from build123d import *

# Parameters (mm, degrees)
SKETCH_1_W      = 29
SKETCH_1_H      = 12.7
EXTRUDE_1_DEPTH = 15.7
EXTRUDE_2_DEPTH = 3.5
FILLET_1_R      = 0.05
CHAMFER_1_SIZE  = 1.5
FILLET_2_R      = 0.75


with BuildPart() as part:
    # Эскиз1 → Бобышка-Вытянуть1 (new body)
    with BuildSketch(Plane(origin=(0, 0, 0), x_dir=(1, 0, 0), z_dir=(0, 1, 0))):
        Rectangle(SKETCH_1_W, SKETCH_1_H)
    extrude(amount=EXTRUDE_1_DEPTH)

    # Эскиз2 → Бобышка-Вытянуть2 (add)
    with BuildSketch(Plane.XZ):
        with BuildLine():
            Line((-12.3, 4.15), (-11.9, 4.15))
            ThreePointArc((-11.9, 4.15), (-11.864644661, 4.135355339), (-11.85, 4.1))
            Line((-11.85, 4.1), (-11.85, 3.4))
            ThreePointArc((-11.85, 3.4), (-11.864644661, 3.364644661), (-11.9, 3.35))
            Line((-11.9, 3.35), (-12.3, 3.35))
            ThreePointArc((-12.3, 3.35), (-12.335355339, 3.364644661), (-12.35, 3.4))
            Line((-12.35, 3.4), (-12.35, 4.1))
            ThreePointArc((-12.35, 4.1), (-12.335355339, 4.135355339), (-12.3, 4.15))
        make_face()
        with BuildLine():
            Line((2.65, 4.1), (2.65, 3.4))
            ThreePointArc((2.65, 3.4), (2.664644661, 3.364644661), (2.7, 3.35))
            Line((2.7, 3.35), (3.1, 3.35))
            ThreePointArc((3.1, 3.35), (3.135355339, 3.364644661), (3.15, 3.4))
            Line((3.15, 3.4), (3.15, 4.1))
            ThreePointArc((3.15, 4.1), (3.135355339, 4.135355339), (3.1, 4.15))
            Line((3.1, 4.15), (2.7, 4.15))
            ThreePointArc((2.7, 4.15), (2.664644661, 4.135355339), (2.65, 4.1))
        make_face()
        with BuildLine():
            Line((7.65, 4.1), (7.65, 3.4))
            ThreePointArc((7.65, 3.4), (7.664644661, 3.364644661), (7.7, 3.35))
            Line((7.7, 3.35), (8.1, 3.35))
            ThreePointArc((8.1, 3.35), (8.135355339, 3.364644661), (8.15, 3.4))
            Line((8.15, 3.4), (8.15, 4.1))
            ThreePointArc((8.15, 4.1), (8.135355339, 4.135355339), (8.1, 4.15))
            Line((8.1, 4.15), (7.7, 4.15))
            ThreePointArc((7.7, 4.15), (7.664644661, 4.135355339), (7.65, 4.1))
        make_face()
        with BuildLine():
            Line((12.65, 4.1), (12.65, 3.4))
            ThreePointArc((12.65, 3.4), (12.664644661, 3.364644661), (12.7, 3.35))
            Line((12.7, 3.35), (13.1, 3.35))
            ThreePointArc((13.1, 3.35), (13.135355339, 3.364644661), (13.15, 3.4))
            Line((13.15, 3.4), (13.15, 4.1))
            ThreePointArc((13.15, 4.1), (13.135355339, 4.135355339), (13.1, 4.15))
            Line((13.1, 4.15), (12.7, 4.15))
            ThreePointArc((12.7, 4.15), (12.664644661, 4.135355339), (12.65, 4.1))
        make_face()
        with BuildLine():
            Line((2.65, -3.4), (2.65, -4.1))
            ThreePointArc((2.65, -4.1), (2.664644661, -4.135355339), (2.7, -4.15))
            Line((2.7, -4.15), (3.1, -4.15))
            ThreePointArc((3.1, -4.15), (3.135355339, -4.135355339), (3.15, -4.1))
            Line((3.15, -4.1), (3.15, -3.4))
            ThreePointArc((3.15, -3.4), (3.135355339, -3.364644661), (3.1, -3.35))
            Line((3.1, -3.35), (2.7, -3.35))
            ThreePointArc((2.7, -3.35), (2.664644661, -3.364644661), (2.65, -3.4))
        make_face()
        with BuildLine():
            Line((7.65, -3.4), (7.65, -4.1))
            ThreePointArc((7.65, -4.1), (7.664644661, -4.135355339), (7.7, -4.15))
            Line((7.7, -4.15), (8.1, -4.15))
            ThreePointArc((8.1, -4.15), (8.135355339, -4.135355339), (8.15, -4.1))
            Line((8.15, -4.1), (8.15, -3.4))
            ThreePointArc((8.15, -3.4), (8.135355339, -3.364644661), (8.1, -3.35))
            Line((8.1, -3.35), (7.7, -3.35))
            ThreePointArc((7.7, -3.35), (7.664644661, -3.364644661), (7.65, -3.4))
        make_face()
        with BuildLine():
            Line((12.65, -3.4), (12.65, -4.1))
            ThreePointArc((12.65, -4.1), (12.664644661, -4.135355339), (12.7, -4.15))
            Line((12.7, -4.15), (13.1, -4.15))
            ThreePointArc((13.1, -4.15), (13.135355339, -4.135355339), (13.15, -4.1))
            Line((13.15, -4.1), (13.15, -3.4))
            ThreePointArc((13.15, -3.4), (13.135355339, -3.364644661), (13.1, -3.35))
            Line((13.1, -3.35), (12.7, -3.35))
            ThreePointArc((12.7, -3.35), (12.664644661, -3.364644661), (12.65, -3.4))
        make_face()
        with BuildLine():
            Line((-12.35, -3.4), (-12.35, -4.1))
            ThreePointArc((-12.35, -4.1), (-12.335355339, -4.135355339), (-12.3, -4.15))
            Line((-12.3, -4.15), (-11.9, -4.15))
            ThreePointArc((-11.9, -4.15), (-11.864644661, -4.135355339), (-11.85, -4.1))
            Line((-11.85, -4.1), (-11.85, -3.4))
            ThreePointArc((-11.85, -3.4), (-11.864644661, -3.364644661), (-11.9, -3.35))
            Line((-11.9, -3.35), (-12.3, -3.35))
            ThreePointArc((-12.3, -3.35), (-12.335355339, -3.364644661), (-12.35, -3.4))
        make_face()
    extrude(amount=EXTRUDE_2_DEPTH)

    # Скругление1
    fillet_1_edges = [part.edges().sort_by_distance(p)[0] for p in [
        (7.664644661, -3.5, -4.135355339),
        (7.9, -3.5, -4.15),
        (8.135355339, -3.5, -4.135355339),
        (8.15, -3.5, -3.75),
        (8.135355339, -3.5, -3.364644661),
        (7.9, -3.5, -3.35),
        (7.664644661, -3.5, -3.364644661),
        (7.65, -3.5, -3.75),
        (12.664644661, -3.5, -4.135355339),
        (12.9, -3.5, -4.15),
        (13.135355339, -3.5, -4.135355339),
        (13.15, -3.5, -3.75),
        (13.135355339, -3.5, -3.364644661),
        (12.9, -3.5, -3.35),
        (12.664644661, -3.5, -3.364644661),
        (12.65, -3.5, -3.75),
        (-12.335355339, -3.5, -4.135355339),
        (-12.1, -3.5, -4.15),
        (-11.864644661, -3.5, -4.135355339),
        (-11.85, -3.5, -3.75),
        (-11.864644661, -3.5, -3.364644661),
        (-12.1, -3.5, -3.35),
        (-12.335355339, -3.5, -3.364644661),
        (-12.35, -3.5, -3.75),
        (-12.335355339, -3.5, 3.364644661),
        (-12.1, -3.5, 3.35),
        (-11.864644661, -3.5, 3.364644661),
        (-11.85, -3.5, 3.75),
        (-11.864644661, -3.5, 4.135355339),
        (-12.1, -3.5, 4.15),
        (-12.335355339, -3.5, 4.135355339),
        (-12.35, -3.5, 3.75),
        (7.664644661, -3.5, 3.364644661),
        (7.9, -3.5, 3.35),
        (8.135355339, -3.5, 3.364644661),
        (8.15, -3.5, 3.75),
        (8.135355339, -3.5, 4.135355339),
        (7.9, -3.5, 4.15),
        (7.664644661, -3.5, 4.135355339),
        (7.65, -3.5, 3.75),
        (12.664644661, -3.5, 3.364644661),
        (12.9, -3.5, 3.35),
        (13.135355339, -3.5, 3.364644661),
        (13.15, -3.5, 3.75),
        (13.135355339, -3.5, 4.135355339),
        (12.9, -3.5, 4.15),
        (12.664644661, -3.5, 4.135355339),
        (12.65, -3.5, 3.75),
    ]]
    fillet(fillet_1_edges, radius=FILLET_1_R)

    # Фаска1
    chamfer_1_edges = [part.edges().sort_by_distance(p)[0] for p in [
        (14.5, 15.7, 0),
    ]]
    chamfer(chamfer_1_edges, length=CHAMFER_1_SIZE)

    # Скругление2
    fillet_2_edges = [part.edges().sort_by_distance(p)[0] for p in [
        (-14.5, 15.7, 0),
        (-0.75, 15.7, 6.35),
        (-0.75, 15.7, -6.35),
        (13, 15.7, 0),
        (14.5, 7.1, -6.35),
        (13.75, 14.95, -6.35),
        (14.5, 7.1, 6.35),
        (14.5, 14.2, 0),
        (13.75, 14.95, 6.35),
        (-14.5, 7.85, 6.35),
        (-14.5, 7.85, -6.35),
    ]]
    fillet(fillet_2_edges, radius=FILLET_2_R)


solid = part.part
Can you work these out from the model? Positions are in its coordinate system, mm. Coordinates: 2 decimals unless noted, no trailing zeros. Write each loop counter-clockwise with the first axis right and the second up, starting at its lowest first coordinate (ties: lowest second). Pieces come first, ordered by that corner, then holes. Notation, with made-up numbers: (-17, 23) -> (40, 23) arc R14 ccw to (40, 38) -> close; hole circle Ø9 at (5.25, 27). An arc over 180 degrees is marked (long way). Write item = value, one per line.
(1) If I drill on probe 1 along Z at (x, y) = (1, 15); probe 2 along Y at (x, z) = (6.5, -4); probe 3 along Y at (x, z) = (-7, -6), over which ranges is the centre line in solid material (lowest first)?
Verdict:
probe_1 = -6.35 to 6.35
probe_2 = 0 to 15.7
probe_3 = 0 to 15.58
(2) Imagine slicing it at C-C (x = -2.75). Please give me the cut outline in (y, z), and give its area (3 significant figures).
Verdict:
outline = (0, -6.35) -> (14.95, -6.35) arc R0.75 ccw to (15.7, -5.6) -> (15.7, 5.6) arc R0.75 ccw to (14.95, 6.35) -> (0, 6.35) -> close
area = 199 mm^2
(3) Imagine slicing it at A-A (y = -2). State how many separate pieces and enclosed holes the cut face has, and give its area (3 significant figures).
Verdict:
separate_pieces = 8
enclosed_holes = 0
area = 3.18 mm^2
(4) Imagine slicing it at B-B (z = -0.5). Please give me the cut outline in (x, y), and give its area (3 significant figures).
Verdict:
outline = (-14.5, 0) -> (14.5, 0) -> (14.5, 13.89) arc R0.75 ccw to (14.28, 14.42) -> (13.22, 15.48) arc R0.75 ccw to (12.69, 15.7) -> (-13.75, 15.7) arc R0.75 ccw to (-14.5, 14.95) -> close
area = 454 mm^2
(5) For pin 1 (3 mm diameter, centred on x = -2, z = 1, fed in from -Y); pin 2 (0.6 mm diameter, centred on y = -2, z = 3.5, fed in from +X); pin 3 (0.6 mm diameter, centred on y = -2, z = -4, fed in from -X), each with a flat end and sliding along its axis, tell me the tip position at first contact or that it passes through.
Verdict:
pin_1 = 0
pin_2 = 13.15
pin_3 = -12.35
